Here's how the part is built. I have some questions about the finished solid (model axes, mm). Face numbers are marked on the shaded views. A direction names the side the tool comes from. Round coordinates to 2 decimals unless told otherwise and drop trailing zeros. Loops run counter-clockwise (first coordinate to the right, second up) from the corner with the lowest first, then second, coordinate; pieces in that order, holes last. Notation, with made-up numbers: M -9.75,50.5 L 44.25,50.5 A21 cw 44.25,62.5 Z; hole C 68.5,6.25 d2. An arc over 180 degrees is marked long. Use a Markdown table: item, result.
from build123d import *

# Parameters (mm, degrees)
SKETCH1_R           = 27
BOSS_EXTRUDE1_DEPTH = 3
SKETCH2_W           = 8
SKETCH2_H           = 3
BOSS_EXTRUDE2_DEPTH = 34
SKETCH5_R           = 0.5
CUT_EXTRUDE1_DEPTH  = 5
FILLET1_R           = 4
SKETCH6_W           = 15
SKETCH6_H           = 3
BOSS_EXTRUDE3_DEPTH = 35
SKETCH7_R           = 1.25
SKETCH7_W           = 12
SKETCH7_H           = 23
CUT_EXTRUDE2_DEPTH  = 5
SKETCH8_W           = 15
SKETCH8_H           = 20
BOSS_EXTRUDE4_DEPTH = 2
SKETCH9_W           = 15
SKETCH9_H           = 37
BOSS_EXTRUDE5_DEPTH = 2
SKETCH10_W          = 10
SKETCH10_H          = 4
BOSS_EXTRUDE6_DEPTH = 28
SKETCH11_R          = 1.5
CUT_EXTRUDE3_DEPTH  = 5
SKETCH12_R          = 1.5
BOSS_EXTRUDE7_DEPTH = 5


with BuildPart() as part:
    # Sketch1 → Boss-Extrude1 (new body)
    with BuildSketch(Plane.XY):
        Circle(SKETCH1_R)
    extrude(amount=BOSS_EXTRUDE1_DEPTH)

    # Sketch2 → Boss-Extrude2 (add)
    with BuildSketch(Plane.XY.offset(3)):
        with Locations((0, 22)):
            Rectangle(SKETCH2_W, SKETCH2_H)
    extrude(amount=BOSS_EXTRUDE2_DEPTH)

    # Sketch5 → Cut-Extrude1 (cut)
    with BuildSketch(Plane(origin=(0, 23.5, 0), x_dir=(1, 0, 0), z_dir=(0, 1, 0))):
        with Locations(Location((0, -6, 0), (0, 0, 270))):
            Circle(SKETCH5_R)
        with Locations(Location((0, -8, 0), (0, 0, 270))):
            Circle(SKETCH5_R)
        with Locations(Location((0, -10, 0), (0, 0, 270))):
            Circle(SKETCH5_R)
        with Locations(Location((0, -12, 0), (0, 0, 270))):
            Circle(SKETCH5_R)
        with Locations(Location((0, -14, 0), (0, 0, 270))):
            Circle(SKETCH5_R)
        with Locations(Location((0, -16, 0), (0, 0, 270))):
            Circle(SKETCH5_R)
        with Locations(Location((0, -34.5, 0), (0, 0, 270))):
            Circle(SKETCH5_R)
        with Locations(Location((0, -32.5, 0), (0, 0, 270))):
            Circle(SKETCH5_R)
        with Locations(Location((0, -30.5, 0), (0, 0, 270))):
            Circle(SKETCH5_R)
        with Locations(Location((0, -28.5, 0), (0, 0, 270))):
            Circle(SKETCH5_R)
        with Locations(Location((0, -26.5, 0), (0, 0, 270))):
            Circle(SKETCH5_R)
        with Locations(Location((0, -24.5, 0), (0, 0, 270))):
            Circle(SKETCH5_R)
    extrude(amount=-CUT_EXTRUDE1_DEPTH, mode=Mode.SUBTRACT)

    # Fillet1
    fillet1_edges = [part.edges().sort_by_distance(p)[0] for p in [
        (-4, 22, 37),
        (4, 22, 37),
    ]]
    fillet(fillet1_edges, radius=FILLET1_R - 0.0001)  # a hair under: the kernel refuses the full size

    # Sketch6 → Boss-Extrude3 (add)
    with BuildSketch(Plane(origin=(0, 0, 0), x_dir=(-1, 0, 0), z_dir=(0, 0, -1))):
        with Locations((0, 2)):
            Rectangle(SKETCH6_W, SKETCH6_H)
    extrude(amount=BOSS_EXTRUDE3_DEPTH)

    # Sketch7 → Cut-Extrude2 (cut)
    with BuildSketch(Plane(origin=(0, 3.5, 0), x_dir=(1, 0, 0), z_dir=(0, 1, 0))):
        with Locations(Location((0, 32, 0), (0, 0, 270))):
            Circle(SKETCH7_R)
        with Locations(Location((0, 3, 0), (0, 0, 270))):
            Circle(SKETCH7_R)
        with Locations((0, 17.5)):
            Rectangle(SKETCH7_W, SKETCH7_H)
    extrude(amount=-CUT_EXTRUDE2_DEPTH, mode=Mode.SUBTRACT)

    # Sketch8 → Boss-Extrude4 (add)
    with BuildSketch(Plane(origin=(0, 0, -35), x_dir=(-1, 0, 0), z_dir=(0, 0, -1))):
        with Locations((0, -6.5)):
            Rectangle(SKETCH8_W, SKETCH8_H)
    extrude(amount=BOSS_EXTRUDE4_DEPTH)

    # Sketch9 → Boss-Extrude5 (add)
    with BuildSketch(Plane.XZ.offset(16.5)):
        with Locations((0, -18.5)):
            Rectangle(SKETCH9_W, SKETCH9_H)
    extrude(amount=BOSS_EXTRUDE5_DEPTH)

    # Sketch10 → Boss-Extrude6 (add)
    with BuildSketch(Plane.XY.offset(3)):
        with Locations((0, -21.5)):
            Rectangle(SKETCH10_W, SKETCH10_H)
    extrude(amount=BOSS_EXTRUDE6_DEPTH)

    # Sketch11 → Cut-Extrude3 (cut)
    with BuildSketch(Plane(origin=(0, -19.5, 0), x_dir=(1, 0, 0), z_dir=(0, 1, 0))):
        with Locations(Location((0, -20.25, 0), (0, 0, 270))):
            Circle(SKETCH11_R)
    extrude(amount=-CUT_EXTRUDE3_DEPTH, mode=Mode.SUBTRACT)

    # Sketch12 → Boss-Extrude7 (add)
    with BuildSketch(Plane.XZ.offset(18.5)):
        with Locations(Location((0, -22.5, 0), (0, 0, 270))):
            Circle(SKETCH12_R)
    extrude(amount=BOSS_EXTRUDE7_DEPTH)


solid = part.part
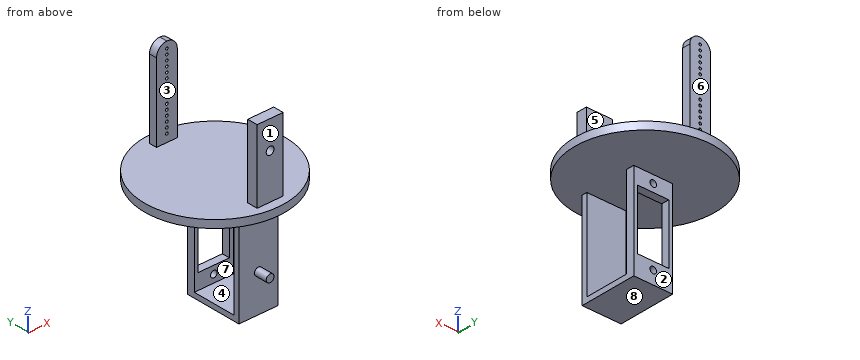
1. I need wall thicknesses on probe 1 along Z at (x, y) = (4.5, 3); probe 2 along X at (y, z) = (22, 14); probe 3 along Y at (x, z) = (6.5, -16.5). Which ranges of each line are inside material? Lowest first, please. Write a range as from..to.
Answer sheet:
| item | result |
|---|---|
| probe 1 | -37..-29, -6..3 |
| probe 2 | -4..-0.5, 0.5..4 |
| probe 3 | -18.5..-16.5, 0.5..3.5 |
2. Which directions (+Z, -Z, +X, -X, +Y, -Y) give clear straight access to the entire face, cutting with the end or side of a thin tool? Please do the marked faces 1, 2, 3 and 4.
Answer sheet:
| item | result |
|---|---|
| face 1 | +Z, +X, -X, -Y |
| face 2 | -Z, +X, -X, +Y |
| face 3 | +Z, +X, -X |
| face 4 | +X, -X |
3. Imagine slicing it at C-C, the plane y = -2.5. Write out the boundary of the cut face in (x, z), then the cut area to 3 significant figures.
Answer sheet:
| item | result |
|---|---|
| outline | M -26.88,0 L 26.88,0 L 26.88,3 L -26.88,3 Z; M -7.5,-37 L 7.5,-37 L 7.5,-35 L -7.5,-35 Z |
| area | 191 mm2 |
4. Imagine slicing it at D-D, the plane x = 19.5. Write out the boundary of the cut face in (y, z).
Answer sheet:
| item | result |
|---|---|
| outline | M -18.67,0 L 18.67,0 L 18.67,3 L -18.67,3 Z |
5. We'd pull the mould along Y, two halves only. Please class the marked faces 5, 6, 7 and 8: +Y half, -Y half, draft (parallel to the pull), parting line (faces both ways), or undercut.
Answer sheet:
| item | result |
|---|---|
| face 5 | undercut |
| face 6 | +Y half |
| face 7 | undercut |
| face 8 | draft |
6. Imagine slicing it at B-B, the plane y = -8. Write out the boundary of the cut face in (x, z), then the cut area to 3 significant figures.
Answer sheet:
| item | result |
|---|---|
| outline | M -25.79,0 L 25.79,0 L 25.79,3 L -25.79,3 Z; M -7.5,-37 L 7.5,-37 L 7.5,-35 L -7.5,-35 Z |
| area | 185 mm2 |
7. For pin 1 Ø3.5 at (x, y) = (-1, 1.5) entering from +Z; pin 2 Ø2 at (y, z) = (-21, 22.5) entering from -X; pin 3 Ø11 at (x, z) = (2, 23.5) entering from +Y, each with a flat end and sliding along its axis, tell me the tip position at first contact or that it passes through.
Answer sheet:
| item | result |
|---|---|
| pin 1 | z = 3 |
| pin 2 | x = -5 |
| pin 3 | y = 23.5 |
8. Imagine slicing it at A-A, the plane z = -3. Write out the boundary of the cut face in (x, y), then the cut area to 3 significant figures.
Answer sheet:
| item | result |
|---|---|
| outline | M -7.5,-18.5 L 7.5,-18.5 L 7.5,-16.5 L -7.5,-16.5 Z; M -7.5,0.5 L -1.25,0.5 L -1.25,3.5 L -7.5,3.5 Z; M 1.25,0.5 L 7.5,0.5 L 7.5,3.5 L 1.25,3.5 Z |
| area | 67.5 mm2 |
